Here's how the part is built. I have some questions about the finished solid (model axes, mm). Give positions to 0.01 mm unless a question says otherwise; leave off trailing zeros. Write each loop counter-clockwise with the first axis right and the second up, starting at its lowest first coordinate (ties: lowest second). Pieces come first, ordered by that corner, then holes. Notation, with made-up numbers: (70, 9.5) - (88, 9.5) arc R33 ccw to (88, 46.5) - close; hole circle Ø9 at (61, 19). An arc over 180 degrees is marked (long way). One line per item, written item: value. Start each with the question number.
1) Imagine slicing it at B-B on z = -81.3. Write out the boundary of the cut face in (x, y), plus the area to 3 significant figures.
2) Imagine slicing it at A-A on z = 0. Write out the boundary of the cut face in (x, y).
3) I'm going to push a flat-ended pin straight in: P1, Ø11.5, axis at x = 0, z = 81.3, coming from the -Y side. Where does the tip first touch, or does it pass through?
4) Imagine slicing it at C-C on x = 0. Write out the boundary of the cut face in (y, z).
5) Imagine slicing it at D-D on y = 11. Count the separate pieces of the cut face and the enclosed holes in it, plus the area to 3 significant figures.
6) Please list where these lines run through material, in increasing order: L1, parallel to X at y = 16, z = 150; L2, parallel to X at y = 23, z = -81.3. Write a range as [from, to].
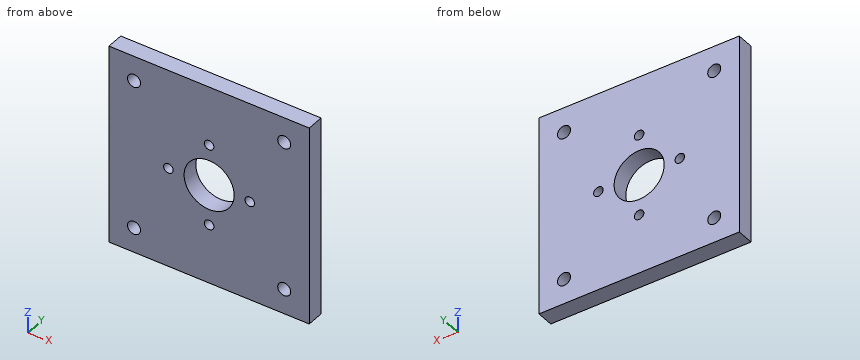
from build123d import *

# Parameters (mm, degrees)
SKETCH1_W           = 400
SKETCH1_H           = 400
SKETCH1_R           = 13
SKETCH1_R_2         = 50
SKETCH1_R_3         = 9.5
BOSS_EXTRUDE1_DEPTH = 34


with BuildPart() as part:
    # Sketch1 → Boss-Extrude1 (new body)
    with BuildSketch(Plane(origin=(0, 0, 0), x_dir=(1, 0, 0), z_dir=(0, 1, 0))):
        Rectangle(SKETCH1_W, SKETCH1_H)
        with Locations((-150, 150)):
            Circle(SKETCH1_R, mode=Mode.SUBTRACT)
        with Locations((-150, -150)):
            Circle(SKETCH1_R, mode=Mode.SUBTRACT)
        with Locations((150, -150)):
            Circle(SKETCH1_R, mode=Mode.SUBTRACT)
        with Locations((150, 150)):
            Circle(SKETCH1_R, mode=Mode.SUBTRACT)
        Circle(SKETCH1_R_2, mode=Mode.SUBTRACT)
        with Locations((0, 81.3)):
            Circle(SKETCH1_R_3, mode=Mode.SUBTRACT)
        with Locations((-81.3, 0)):
            Circle(SKETCH1_R_3, mode=Mode.SUBTRACT)
        with Locations((0, -81.3)):
            Circle(SKETCH1_R_3, mode=Mode.SUBTRACT)
        with Locations((81.3, 0)):
            Circle(SKETCH1_R_3, mode=Mode.SUBTRACT)
    extrude(amount=BOSS_EXTRUDE1_DEPTH)


solid = part.part
Numbers:
1. outline: (-200, 0) - (-9.5, 0) - (-9.5, 34) - (-200, 34) - close; (9.5, 0) - (200, 0) - (200, 34) - (9.5, 34) - close
1. area: 13,000 mm^2
2. outline: (-200, 0) - (-90.8, 0) - (-90.8, 34) - (-200, 34) - close; (-71.8, 0) - (-50, 0) - (-50, 34) - (-71.8, 34) - close; (50, 0) - (71.8, 0) - (71.8, 34) - (50, 34) - close; (90.8, 0) - (200, 0) - (200, 34) - (90.8, 34) - close
3. P1: through
4. outline: (0, -200) - (34, -200) - (34, -90.8) - (0, -90.8) - close; (0, -71.8) - (34, -71.8) - (34, -50) - (0, -50) - close; (0, 50) - (34, 50) - (34, 71.8) - (0, 71.8) - close; (0, 90.8) - (34, 90.8) - (34, 200) - (0, 200) - close
5. separate pieces: 1
5. enclosed holes: 9
5. area: 149,000 mm^2
6. L1: [-200, -163], [-137, 137], [163, 200]
6. L2: [-200, -9.5], [9.5, 200]
